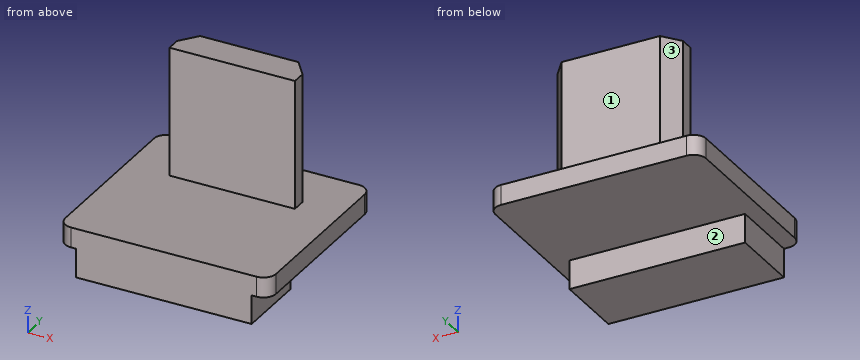
```python
from build123d import *

# Parameters (mm, degrees)
SKETCH_W     = 16.8
SKETCH_H     = 15
PAD_DEPTH    = 1.6
FILLET_R     = 1
SKETCH001_W  = 10
SKETCH001_H  = 2.5
PAD001_DEPTH = 10.26
POCKET_DEPTH = 10.26
SKETCH003_W  = 14
SKETCH003_H  = 5.7
PAD002_DEPTH = 2.3


with BuildPart() as part:
    # Sketch → Pad (new body)
    with BuildSketch(Plane.XY):
        Rectangle(SKETCH_W, SKETCH_H)
    extrude(amount=PAD_DEPTH)

    # Fillet
    fillet_edges = [part.edges().sort_by_distance(p)[0] for p in [
        (8.4, 7.5, 0.8),
        (8.4, -7.5, 0.8),
        (-8.4, -7.5, 0.8),
        (-8.4, 7.5, 0.8),
    ]]
    fillet(fillet_edges, radius=FILLET_R)

    # Sketch001 (on Face5 of Fillet) → Pad001 (join)
    with BuildSketch(Plane.XY.offset(1.6)):
        with Locations((0.1, 3.59)):
            Rectangle(SKETCH001_W, SKETCH001_H)
    extrude(amount=PAD001_DEPTH)

    # Sketch002 (on Face15 of Pad001) → Pocket (cut)
    with BuildSketch(Plane.XY.offset(11.86)):
        Polygon((-4.9, 3.44), (-4.9, 4.84), (-3.82, 4.84), align=None)
        Polygon((5.1, 4.84), (4.02, 4.84), (5.1, 3.44), align=None)
    extrude(amount=-POCKET_DEPTH, mode=Mode.SUBTRACT)

    # Sketch003 (on Face2 of Pocket) → Pad002 (join)
    with BuildSketch(Plane(origin=(0, 0, 0), x_dir=(1, 0, 0), z_dir=(0, 0, -1))):
        with Locations((0, 4.65)):
            Rectangle(SKETCH003_W, SKETCH003_H)
    extrude(amount=PAD002_DEPTH)


solid = part.part
```
Design review of the part built by this model. Coordinates are the model's own, in mm. Face numbers are marked on the shaded views. A direction names the side the tool comes from. Coordinates: 2 decimals unless noted, no trailing zeros. Write each loop counter-clockwise with the first axis right and the second up, starting at its lowest first coordinate (ties: lowest second). Pieces come first, ordered by that corner, then holes. Notation, with made-up numbers: M -23,-4 L -1,-4 A27 cw -1,24 Z; hole C -5.5,89.5 d11. An arc over 180 degrees is marked long. Answer as a JSON object with one key per item and string values.
Item 1: Wall thickness on probe 1 along Y at (x, z) = (0.25, 9.5); probe 2 along Z at (x, y) = (7.75, -5.5); probe 3 along X at (y, z) = (-6, -0.75): over which ranges is each line inside the solid? List them lowest first.
Outcome:
{"probe 1": "2.34 to 4.84", "probe 2": "0 to 1.6", "probe 3": "-7 to 7"}
Item 2: Add section B-B, the plane z = 3.5. Give the boundary of the cut face in (x, y).
Outcome:
{"outline": "M -4.9,2.34 L 5.1,2.34 L 5.1,3.44 L 4.02,4.84 L -3.82,4.84 L -4.9,3.44 Z"}
Item 3: Machinability: for the marked faces 1, 2 and 3, which of the approach directions +Z, -Z, +X, -X, +Y, -Y give a long, thin tool a straight path to every point of the face, cutting with its end or side? Answer none if there is none.
Outcome:
{"face 1": "+Z, +X, -X, +Y", "face 2": "-Z, +X, -X, +Y", "face 3": "+Z, -X, +Y"}
Item 4: Insertion check: pin 1 Ø1.2 at (y, z) = (-3.5, -1.5) entering from -X; pin 2 Ø5 at (x, z) = (2, 6) entering from -Y; pin 3 Ø0.9 at (y, z) = (3, 5) entering from -X. Each pin has a flat end and moves straight along its axis. Give the tip position at first contact, or say it passes through.
Outcome:
{"pin 1": "x = -7", "pin 2": "y = 2.34", "pin 3": "x = -4.9"}
Item 5: Add section C-C, the plane y = -2.25. Give the boundary of the cut face in (x, z).
Outcome:
{"outline": "M -8.4,0 L -7,0 L -7,-2.3 L 7,-2.3 L 7,0 L 8.4,0 L 8.4,1.6 L -8.4,1.6 Z"}
Item 6: Add section D-D, the plane y = 3.75. Give the boundary of the cut face in (x, z), and give its area (3 significant figures).
Outcome:
{"outline": "M -8.4,0 L 8.4,0 L 8.4,1.6 L 4.86,1.6 L 4.86,11.86 L -4.66,11.86 L -4.66,1.6 L -8.4,1.6 Z", "area": "125 mm²"}
Item 7: Add section A-A, the plane x = -3.5. Give the boundary of the cut face in (y, z).
Outcome:
{"outline": "M -7.5,-2.3 L -1.8,-2.3 L -1.8,0 L 7.5,0 L 7.5,1.6 L 4.84,1.6 L 4.84,11.86 L 2.34,11.86 L 2.34,1.6 L -7.5,1.6 Z"}
